The model under review builds one solid part; all positions refer to its coordinate system, in mm. Face numbers are marked on the shaded views. A direction names the side the tool comes from. Round coordinates to 2 decimals unless told otherwise and drop trailing zeros. Loops run counter-clockwise (first coordinate to the right, second up) from the corner with the lowest first, then second, coordinate; pieces in that order, holes last. Notation, with made-up numbers: M -8.5,53 L 21.5,53 A16 ccw 21.5,78 Z; hole C 8.25,72.5 d5. An arc over 180 degrees is marked long. Answer in a Markdown table with one row per item. Add a question column.
from build123d import *

# Parameters (mm, degrees)
AUFSATZ_LINEAR_AUSTRAGEN1_DEPTH = 10
SKIZZE2_R                       = 1.75
SCHNITT_LINEAR_AUSTRAGEN1_DEPTH = 36.05
SKIZZE4_R                       = 2.25
SCHNITT_LINEAR_AUSTRAGEN3_DEPTH = 50.25
VERRUNDUNG1_R                   = 10
SKIZZE5_W                       = 5.55
SKIZZE5_H                       = 5.55
SCHNITT_LINEAR_AUSTRAGEN4_DEPTH = 2
SCHNITT_LINEAR_AUSTRAGEN5_DEPTH = 11
FASE1_SIZE                      = 1.5
SCHNITT_LINEAR_AUSTRAGEN6_DEPTH = 11


with BuildPart() as part:
    # Skizze1 → Aufsatz-Linear austragen1 (new body)
    with BuildSketch(Plane.XY):
        with BuildLine():
            Line((0.5, -26.545291485), (0.5, -30.545908073))
            Line((0.5, -30.545908073), (0.5, -37.545908073))
            Line((0.5, -37.545908073), (4.5, -37.545908073))
            Line((4.5, -37.545908073), (4.5, -30.216758595))
            ThreePointArc((4.5, -30.216758595), (29.558680329, -7.719256261), (18.7, 24.158073185))
            Line((18.7, 24.158073185), (18.7, 51.55))
            Line((18.7, 51.55), (10.2, 51.55))
            Line((10.2, 51.55), (10.2, 31.55))
            Line((10.2, 31.55), (-10.2, 31.55))
            Line((-10.2, 31.55), (-10.2, 51.55))
            Line((-10.2, 51.55), (-18.7, 51.55))
            Line((-18.7, 51.55), (-18.7, 24.158073185))
            ThreePointArc((-18.7, 24.158073185), (-29.558680329, -7.719256261), (-4.5, -30.216758595))
            Line((-4.5, -30.216758595), (-4.5, -37.545908073))
            Line((-4.5, -37.545908073), (-0.5, -37.545908073))
            Line((-0.5, -37.545908073), (-0.5, -30.545908073))
            Line((-0.5, -30.545908073), (-0.5, -26.545291485))
            ThreePointArc((-0.5, -26.545291485), (0, 26.55), (0.5, -26.545291485))
        make_face()
    extrude(amount=AUFSATZ_LINEAR_AUSTRAGEN1_DEPTH)

    # Skizze2 → Schnitt-Linear austragen1 (cut, through all)
    with BuildSketch(Plane.ZY.offset(4.5)):
        with Locations((5, -33.881333334)):
            Circle(SKIZZE2_R)
    extrude(amount=-SCHNITT_LINEAR_AUSTRAGEN1_DEPTH, mode=Mode.SUBTRACT)

    # Skizze4 → Schnitt-Linear austragen3 (cut, through all)
    with BuildSketch(Plane.ZY.offset(18.7)):
        with Locations((5, 41.55)):
            Circle(SKIZZE4_R)
    extrude(amount=-SCHNITT_LINEAR_AUSTRAGEN3_DEPTH, mode=Mode.SUBTRACT)

    # Verrundung1
    verrundung1_edges = [part.edges().sort_by_distance(p)[0] for p in [
        (-18.7, 24.158073185, 5),
        (18.7, 24.158073185, 5),
    ]]
    fillet(verrundung1_edges, radius=VERRUNDUNG1_R)

    # Skizze5 → Schnitt-Linear austragen4 (cut)
    with BuildSketch(Plane.ZY.offset(4.5)):
        with Locations((5, -33.881333334)):
            Rectangle(SKIZZE5_W, SKIZZE5_H)
    extrude(amount=-SCHNITT_LINEAR_AUSTRAGEN4_DEPTH, mode=Mode.SUBTRACT)

    # Skizze6 → Schnitt-Linear austragen5 (cut, through all)
    with BuildSketch(Plane.XY):
        Polygon((0, 0), (0, 63.91348789), (40.013946788, 63.91348789), (48.360414216, -54.819102682), (0, -54.819102682), align=None)
    extrude(amount=SCHNITT_LINEAR_AUSTRAGEN5_DEPTH, mode=Mode.SUBTRACT)

    # Fase1
    fase1_edges = [part.edges().sort_by_distance(p)[0] for p in [
        (-18.7, 40.098167422, 0),
        (-18.7, 40.098167422, 10),
        (-29.006358008, -9.588206043, 0),
        (-29.006358008, -9.588206043, 10),
        (-19.459415096, 24.823823807, 0),
        (-19.459415096, 24.823823807, 10),
    ]]
    chamfer(fase1_edges, length=FASE1_SIZE)

    # Skizze7 → Schnitt-Linear austragen6 (cut, through all)
    with BuildSketch(Plane.XY.offset(10)):
        Polygon((1.325, 29.05), (0, 29.05), (0, 31.55), (-0.15, 31.55), (-0.15, 29.05), (-1.325, 29.05), (-1.325, 23.522445011), (1.325, 23.522445011), align=None)
    extrude(amount=-SCHNITT_LINEAR_AUSTRAGEN6_DEPTH, mode=Mode.SUBTRACT)


solid = part.part
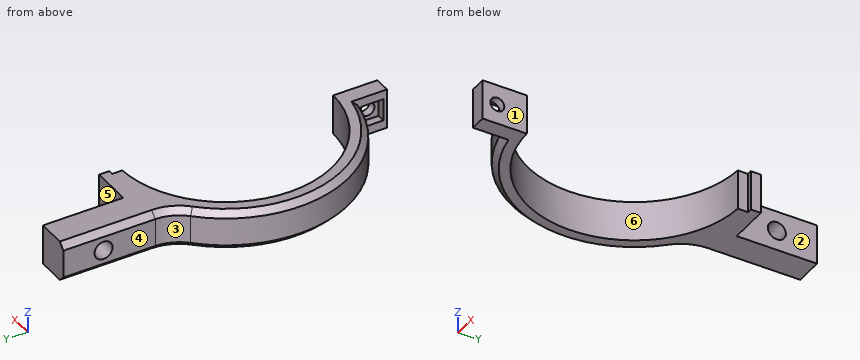
1. To check wall thickness, follow probe 1 along Y at (x, z) = (-1, 5); probe 2 along Y at (x, z) = (-12.25, 5); probe 3 along X at (y, z) = (29, 5.75) (3 decimals). State the ranges of each line that lie inside material, in increasing order.
2. Take a section at B-B, the plane y = 41.55. State the section outline as (x, z) points, and give its area (3 significant figures).
3. For pin 1 Ø2 at (x, z) = (-14.5, 1.5) entering from -Y; pin 2 Ø1.5 at (y, z) = (6.5, 2.5) entering from -X; pin 3 Ø2 at (x, z) = (-23.5, 1.5) entering from +Y; pin 4 Ø6 at (x, y) = (-15, 20.5) entering from -Z, all flat-tipped, find the tip position at first contact; note any pin that passes through.
4. Machinability: for the marked faces 1, 2 and 3, which of the approach directions +Z, -Z, +X, -X, +Y, -Y give a long, thin tool a straight path to every point of the face, cutting with its end or side? Answer none if there is none.
5. Take a section at D-D, the plane x = -13.5. State how many separate pieces and enclosed holes the cut face has, and give its area (3 significant figures).
6. Mouldability with a two-part tool opening along Y and no side actions: class the marked faces 4, 5 and 6 as released by +Y, released by -Y, zero draft, split by the parting line, or undercut.
7. Take a section at A-A, the plane z = 5. State the section outline as (x, y) points (3 decimals).
8. Take a section at C-C, the plane y = 0. State the section outline as (x, z) points.
Check sheet entries:
| question | item | result |
|---|---|---|
| 1 | probe 1 | y = -37.55 to -35.63, -32.13 to -26.53, 29.05 to 31.55 |
| 1 | probe 2 | y = -27.99 to -23.56, 23.56 to 39.3, 43.8 to 51.55 |
| 1 | probe 3 | x = -18.7 to -1.325 |
| 2 | outline | M -18.7,1.5 L -17.2,0 L -10.2,0 L -10.2,2.75 L -18.7,2.75 Z; M -18.7,7.25 L -10.2,7.25 L -10.2,10 L -17.2,10 L -18.7,8.5 Z |
| 2 | area | 44.5 mm^2 |
| 3 | pin 1 | stops at y = -27.41 |
| 3 | pin 2 | stops at x = -30 |
| 3 | pin 3 | stops at y = 20.67 |
| 3 | pin 4 | stops at z = 0 |
| 4 | face 1 | +Z, -Z, +X, -Y |
| 4 | face 2 | +Z, -Z, +X, +Y |
| 4 | face 3 | +Z, -Z, -X, +Y |
| 5 | separate pieces | 2 |
| 5 | enclosed holes | 1 |
| 5 | area | 314 mm^2 |
| 6 | face 4 | zero draft |
| 6 | face 5 | released by +Y |
| 6 | face 6 | undercut |
| 7 | outline | M -21.622,21.582 A30.55 ccw -4.5,-30.217 L -4.5,-31.106 L -2.5,-31.106 L -2.5,-32.131 L -0.5,-32.131 L -0.5,-26.545 A26.55 cw -1.325,26.517 L -1.325,29.05 L -0.15,29.05 L -0.15,31.55 L -10.2,31.55 L -10.2,39.3 L -18.7,39.3 L -18.7,28.646 A10 cw Z; M -18.7,43.8 L -10.2,43.8 L -10.2,51.55 L -18.7,51.55 Z; M -4.5,-37.546 L -0.5,-37.546 L -0.5,-35.631 L -2.5,-35.631 L -2.5,-36.656 L -4.5,-36.656 Z |
| 8 | outline | M -30.55,1.5 L -29.05,0 L -26.55,0 L -26.55,10 L -29.05,10 L -30.55,8.5 Z |
